from build123d import *

# Parameters (mm, degrees)
BOX001_W     = 10
BOX001_H     = 10
BOX001_DEPTH = 10
BOX_W        = 10
BOX_H        = 14
BOX_DEPTH    = 14


with BuildPart() as box001:
    # Box001 → Box001 (new body)
    with BuildSketch(Plane(origin=(10, 0, 0), x_dir=(1, 0, 0), z_dir=(0, 0, 1))):
        with Locations((5, 5)):
            Rectangle(BOX001_W, BOX001_H)
    extrude(amount=BOX001_DEPTH)


with BuildPart() as obj1:
    # Box → Box (new body)
    with BuildSketch(Plane.XY):
        with Locations((5, 7)):
            Rectangle(BOX_W, BOX_H)
    extrude(amount=BOX_DEPTH)

    # Fusion: union Box001
    add(box001.part)


solid = obj1.part
Design review of the part built by this model. Coordinates are the model's own, in mm. A direction names the side the tool comes from. Coordinates: 2 decimals unless noted, no trailing zeros. Order: outer loops, then holes, each group sorted by start corner. A loop starts at its lowest first (then second) coordinate and runs counter-clockwise, first axis right, second up. Notation, with made-up numbers: (87.5, 25.25) -> (138.5, 25.25) arc R27 ccw to (138.5, 55.25) -> close; hole circle Ø11 at (48.25, 50). An arc over 180 degrees is marked (long way). One line per item, written item: value.
1) We need section D-D, the plane y = 11.5. Give the boundary of the cut face in (x, z).
Output values:
outline: (0, 0) -> (10, 0) -> (10, 14) -> (0, 14) -> close
2) Clearance check with flat-ended pins moving along their axes: P1, Ø2, axis at y = 8.5, z = 12.5, coming from the +X side; P2, Ø1.5, axis at x = 12, z = 4.5, coming from the +Y side. State where each tip first meets the part, or that it passes through.
Output values:
P1: stops at x = 10
P2: stops at y = 10
3) Machinability: for faces 1 (the face through (0, 7, 7)), 2 (the face through (15, 5, 10)), 3 (the face through (15, 10, 5)), which of the approach directions +Z, -Z, +X, -X, +Y, -Y give a long, thin tool a straight path to every point of the face, cutting with its end or side? Answer none if there is none.
Output values:
face 1: +Z, -Z, -X, +Y, -Y
face 2: +Z, +X, +Y, -Y
face 3: +Z, -Z, +X, +Y
4) We need section C-C, the plane x = 11. Give the boundary of the cut face in (y, z).
Output values:
outline: (0, 0) -> (10, 0) -> (10, 10) -> (0, 10) -> close
5) To check wall thickness, follow probe 1 along Z at (x, y) = (11.5, 6). State the ranges of the line that lie inside material, in increasing order. Write a range as [from, to].
Output values:
probe 1: z = [0, 10]
6) We need section A-A, the plane y = 4.25. Give the boundary of the cut face in (x, z).
Output values:
outline: (0, 0) -> (20, 0) -> (20, 10) -> (10, 10) -> (10, 14) -> (0, 14) -> close
